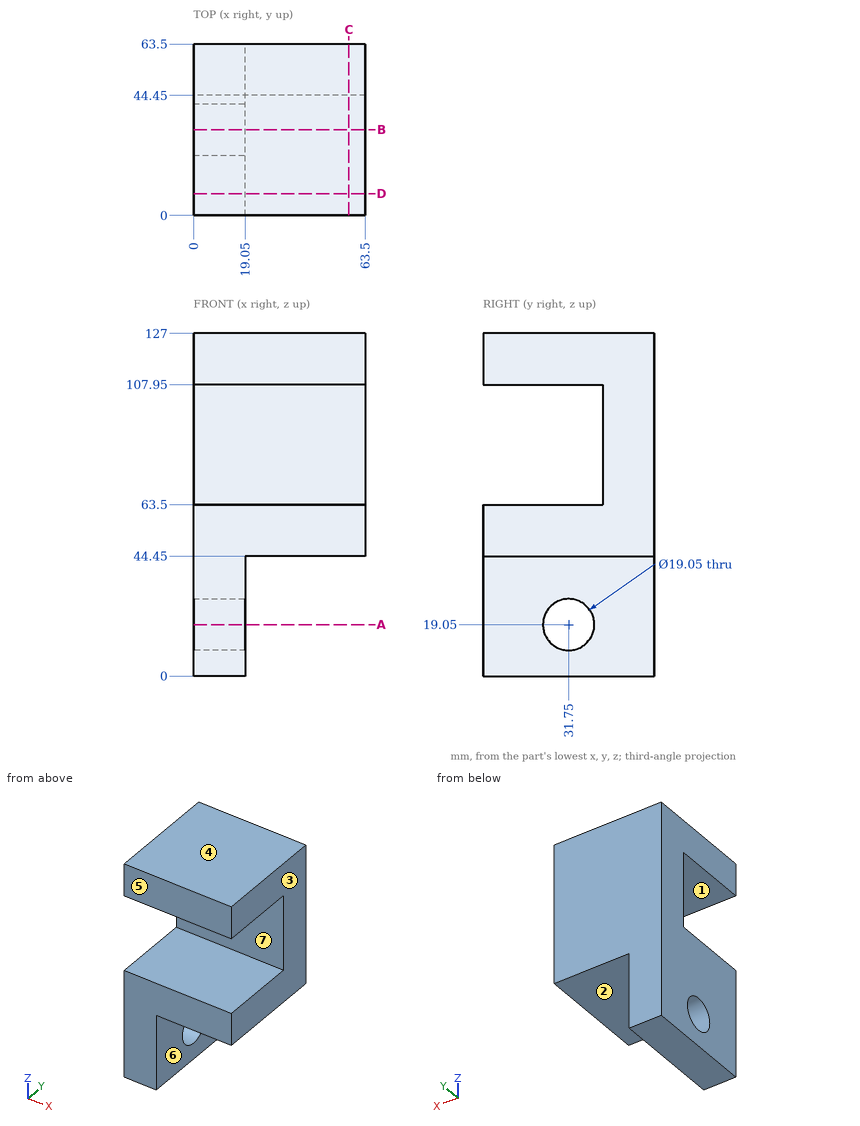
Source: three-view drawing plus pictorial views. Frame: mm from the lowest corner of the part. A direction names the side the tool comes from. Give positions to 0.01 mm unless a question says otherwise; leave off trailing zeros. Write each loop counter-clockwise with the first axis right and the second up, starting at its lowest first coordinate (ties: lowest second). Pieces come first, ordered by that corner, then holes. Notation, with made-up numbers: (-27, 17.25) -> (19, 17.25) arc R24 cw to (19, 27.25) -> close; hole circle Ø1 at (28, 56). An arc over 180 degrees is marked (long way). Write item = value, one per line.
Q1. Cut plane B-B on y = 31.75. Return loops of the section in (x, z) (3 decimals), then the cut area to 3 significant figures.
Here are the results:
outline = (0, 0) -> (19.05, 0) -> (19.05, 9.525) -> (0, 9.525) -> close; (0, 28.575) -> (19.05, 28.575) -> (19.05, 44.45) -> (63.5, 44.45) -> (63.5, 63.5) -> (0, 63.5) -> close; (0, 107.95) -> (63.5, 107.95) -> (63.5, 127) -> (0, 127) -> close
area = 2,900 mm²
Q2. Cut plane D-D on y = 8. Return loops of the section in (x, z).
Here are the results:
outline = (0, 0) -> (19.05, 0) -> (19.05, 44.45) -> (63.5, 44.45) -> (63.5, 63.5) -> (0, 63.5) -> close; (0, 107.95) -> (63.5, 107.95) -> (63.5, 127) -> (0, 127) -> close
Q3. Line query: line 1 (Z direction, x = 12, y = 31); line 2 (Z direction, x = 7, y = 7); line 3 (Z direction, x = 44.5, y = 37). Output: solid intervals per line, ascending. Write a range as from..to.
Here are the results:
line_1 = 0..9.55, 28.55..63.5, 107.95..127
line_2 = 0..63.5, 107.95..127
line_3 = 44.45..63.5, 107.95..127
Q4. Mould query, pull axis Z, two halves, no side actions, for the marked faces 1, 2, 3 and 4. Classes: +Z half, -Z half, draft (parallel to the pull), parting line (faces both ways), or undercut.
Here are the results:
face_1 = undercut
face_2 = -Z half
face_3 = draft
face_4 = +Z half
Q5. Cut plane C-C on x = 57.5. Return loops of the section in (y, z).
Here are the results:
outline = (0, 44.45) -> (63.5, 44.45) -> (63.5, 127) -> (0, 127) -> (0, 107.95) -> (44.45, 107.95) -> (44.45, 63.5) -> (0, 63.5) -> close
Q6. Cut plane A-A on z = 19.05. Return loops of the section in (x, y) (3 decimals).
Here are the results:
outline = (0, 0) -> (19.05, 0) -> (19.05, 22.225) -> (0, 22.225) -> close; (0, 41.275) -> (19.05, 41.275) -> (19.05, 63.5) -> (0, 63.5) -> close
Q7. Reachability of the marked faces 5, 6 and 7 from +Z, -Z, +X, -X, +Y, -Y: full face, straight path, thin tool, end or side. Return the list, or none.
Here are the results:
face_5 = +Z, -Z, +X, -X, -Y
face_6 = -Z, +X, +Y, -Y
face_7 = +X, -X, -Y
